```python
from build123d import *

# Parameters (mm, degrees)
SKETCH_1_R          = 12.5
EXTRUDE_1_DEPTH     = 4
SKETCH_2_R          = 8
EXTRUDE_2_DEPTH     = 10
SKETCH_3_R          = 2.5
CUT_EXTRUDE_1_DEPTH = 23.549944568
SKETCH_4_R          = 6
CUT_EXTRUDE_2_DEPTH = 8
CUT_EXTRUDE_START   = -5
SKETCH_5_R          = 6
CUT_EXTRUDE_3_DEPTH = 5


with BuildPart() as part:
    # 草图1 → 凸台-拉伸1 (new body)
    with BuildSketch(Plane.XY):
        Circle(SKETCH_1_R)
    extrude(amount=EXTRUDE_1_DEPTH)

    # 草图2 → 凸台-拉伸2 (add)
    with BuildSketch(Plane.XY.offset(4)):
        Circle(SKETCH_2_R)
    extrude(amount=EXTRUDE_2_DEPTH)

    # 草图3 → 切除-拉伸1 (cut, through all)
    with BuildSketch(Plane.XY.offset(14)):
        Circle(SKETCH_3_R)
    extrude(amount=-CUT_EXTRUDE_1_DEPTH, mode=Mode.SUBTRACT)

    # 草图4 → 切除-拉伸2 (cut)
    with BuildSketch(Plane.XY.offset(14)):
        Circle(SKETCH_4_R)
    extrude(amount=-CUT_EXTRUDE_2_DEPTH, mode=Mode.SUBTRACT)

    # 草图5 → 切除-拉伸3 (cut)
    with BuildSketch(Plane(origin=(0, 0, 0), x_dir=(-1, 0, 0), z_dir=(0, 0, -1)).offset(CUT_EXTRUDE_START)):
        with Locations(Location((0, 0, 0), (0, 0, 180))):
            Circle(SKETCH_5_R)
    extrude(amount=CUT_EXTRUDE_3_DEPTH, mode=Mode.SUBTRACT)


solid = part.part
```
Can you work these out from the model? Positions are in its coordinate system, mm. A direction names the side the tool comes from. Round coordinates to 2 decimals unless told otherwise and drop trailing zeros. Order: outer loops, then holes, each group sorted by start corner. A loop starts at its lowest first (then second) coordinate and runs counter-clockwise, first axis right, second up. Notation, with made-up numbers: (86, 54.25) -> (96, 54.25) arc R18 cw to (96, 86.25) -> close; hole circle Ø3 at (41.25, 11.25). An arc over 180 degrees is marked (long way). Return JSON: item names as keys, results as strings. Group by question number.
1. If we section it at A-A, the plane x = 0: Write out the boundary of the cut face in (y, z), then the cut area to 3 significant figures.
2. Which directions (+Z, -Z, +X, -X, +Y, -Y) give clear straight access to the entire face, cutting with the end or side of a thin tool? Please do faces 1 (the face through (-0.2, -8.2, 4)), 2 (the face through (5.723, -1.802, 2.535)), 3 (the face through (-0.54, -2.44, 5.51)).
3. If we section it at C-C, the plane x = 4.5: Write out the boundary of the cut face in (y, z), then the cut area to 3 significant figures.
4. We'd pull the mould along X, two halves only. Please class faces 4 (the face through (3, 0, 5)), 5 (the face through (11.923, 3.755, 1.972)), 6 (the face through (-2, 6, 14)): released by +X, released by -X, zero draft, split by the parting line, or undercut.
5. If we section it at D-D, the plane z = 2.25: Write out the boundary of the cut face in (x, y).
6. Will these pins go through, and if not, where does the flat tip stop? pin 1 (3 mm diameter, centred on x = -1, z = 7, fed in from -Y); pin 2 (9.5 mm diameter, centred on x = -2, y = 0.5, fed in from +Z); pin 3 (3 mm diameter, centred on x = 5.5, z = 2.5, fed in from +Y); pin 4 (1 mm diameter, centred on y = 5, z = 9, fed in from -X).
7. I need wall thicknesses on line 1 (Y direction, x = 0, z = 1.4); line 2 (Y direction, x = 0, z = 5.3); line 3 (X direction, y = -2.25, z = 11). Which ranges of each line are inside material? Lowest first, please. Write a range as [from, to].
Output values:
{
 "1": {"outline": "(-12.5, 0) -> (-6, 0) -> (-6, 5) -> (-2.5, 5) -> (-2.5, 6) -> (-6, 6) -> (-6, 14) -> (-8, 14) -> (-8, 4) -> (-12.5, 4) -> close; (2.5, 5) -> (6, 5) -> (6, 0) -> (12.5, 0) -> (12.5, 4) -> (8, 4) -> (8, 14) -> (6, 14) -> (6, 6) -> (2.5, 6) -> close", "area": "99.0 mm²"},
 "2": {"face 1": "+Z", "face 2": "-Z", "face 3": "+Z, -Z"},
 "3": {"outline": "(-11.66, 0) -> (-3.97, 0) -> (-3.97, 5) -> (3.97, 5) -> (3.97, 0) -> (11.66, 0) -> (11.66, 4) -> (6.61, 4) -> (6.61, 14) -> (3.97, 14) -> (3.97, 6) -> (-3.97, 6) -> (-3.97, 14) -> (-6.61, 14) -> (-6.61, 4) -> (-11.66, 4) -> close", "area": "122 mm²"},
 "4": {"face 4": "undercut", "face 5": "split by the parting line", "face 6": "zero draft"},
 "5": {"outline": "circle Ø25 at (0, 0); hole circle Ø12 at (0, 0)"},
 "6": {"pin 1": "y = -8", "pin 2": "z = 14", "pin 3": "y = 11.84", "pin 4": "x = -6.61"},
 "7": {"line 1": "[-12.5, -6], [6, 12.5]", "line 2": "[-8, -2.5], [2.5, 8]", "line 3": "[-7.68, -5.56], [5.56, 7.68]"}
}
